```python
from build123d import *

# Parameters (mm, degrees)
SKETCH1_R          = 2.667
SKETCH1_R_2        = 3.3782
BASE_FLANGE1_DEPTH = 3.175
CHAMFER2_SIZE      = 3.175
EDGE_FLANGE1_DEPTH = 38.1
CHAMFER3_SIZE      = 3.175
SKETCH9_R          = 1.905
CUT_EXTRUDE1_DEPTH = 282.707277995
CUT_EXTRUDE2_DEPTH = 283.261385688
CUT_EXTRUDE3_DEPTH = 283.261385688


# Sheet-metal steps are written as plain solids
with BuildPart() as part:
    # Sketch1 → Base-Flange1 (new body)
    with BuildSketch(Plane(origin=(0, 0, 0), x_dir=(1, 0, 0), z_dir=(0, 1, 0))):
        Polygon((25.4, 0), (0, 0), (0, 132.588), (241.3, 132.588), (241.3, 0), (215.9, 0), (215.9, 21.463), (212.725, 24.638), (212.725, 107.188), (28.575, 107.188), (28.575, 24.638), (25.4, 21.463), align=None)
        with Locations(Location((6.35, 12.7, 0), (0, 0, 270))):
            Circle(SKETCH1_R, mode=Mode.SUBTRACT)
        with Locations(Location((19.05, 12.7, 0), (0, 0, 270))):
            Circle(SKETCH1_R, mode=Mode.SUBTRACT)
        with Locations(Location((222.25, 12.7, 0), (0, 0, 90))):
            Circle(SKETCH1_R, mode=Mode.SUBTRACT)
        with Locations(Location((234.95, 12.7, 0), (0, 0, 90))):
            Circle(SKETCH1_R, mode=Mode.SUBTRACT)
        with Locations(Location((69.85, 114.3, 0), (0, 0, 270))):
            Circle(SKETCH1_R_2, mode=Mode.SUBTRACT)
        with Locations(Location((171.45, 114.3, 0), (0, 0, 90))):
            Circle(SKETCH1_R_2, mode=Mode.SUBTRACT)
    extrude(amount=BASE_FLANGE1_DEPTH)

    # Chamfer2
    chamfer2_edges = [part.edges().sort_by_distance(p)[0] for p in [
        (0, 1.5875, -132.588),
        (241.3, 1.5875, -132.588),
        (241.3, 1.5875, 0),
        (215.9, 1.5875, 0),
        (212.725, 1.5875, -107.188),
        (28.575, 1.5875, -107.188),
        (25.4, 1.5875, 0),
        (0, 1.5875, 0),
    ]]
    chamfer(chamfer2_edges, length=CHAMFER2_SIZE)

    # Edge-Flange1 section (across the edge) → Edge-Flange1 (add)
    with BuildSketch(Plane(origin=(101.6, 0, -134.1755), x_dir=(0, 0, 1), z_dir=(1, 0, 0))):
        with BuildLine():
            Line((-3.175, 1.5875), (-3.175, 47.625))
            Line((-3.175, 47.625), (0, 47.625))
            Line((0, 47.625), (0, 1.5875))
            ThreePointArc((0, 1.5875), (0.464967985, 0.464967985), (1.5875, 0))
            Line((1.5875, 0), (1.5875, -3.175))
            ThreePointArc((1.5875, -3.175), (-1.780096045, -1.780096045), (-3.175, 1.5875))
        make_face()
    extrude(amount=EDGE_FLANGE1_DEPTH)

    # Chamfer3
    chamfer3_edges = [part.edges().sort_by_distance(p)[0] for p in [
        (101.6, -47.625, -135.763),
        (139.7, -47.625, -135.763),
    ]]
    chamfer(chamfer3_edges, length=CHAMFER3_SIZE)

    # Sketch9 → Cut-Extrude1 (cut, through all)
    with BuildSketch(Plane(origin=(0, 0, -137.3505), x_dir=(-1, 0, 0), z_dir=(0, 0, -1))):
        with Locations(Location((-120.65, -38.989, 0), (0, 0, 90))):
            Circle(SKETCH9_R)
        with Locations(Location((-120.65, -19.939, 0), (0, 0, 90))):
            Circle(SKETCH9_R)
    extrude(amount=-CUT_EXTRUDE1_DEPTH, mode=Mode.SUBTRACT)

    # Sketch10 → Cut-Extrude2 (cut, through all)
    with BuildSketch(Plane(origin=(0, 3.175, 0), x_dir=(1, 0, 0), z_dir=(0, 1, 0))):
        with BuildLine():
            Line((115.8875, 127.8255), (125.4125, 127.8255))
            ThreePointArc((125.4125, 127.8255), (127, 126.238), (125.4125, 124.6505))
            Line((125.4125, 124.6505), (115.8875, 124.6505))
            ThreePointArc((115.8875, 124.6505), (114.3, 126.238), (115.8875, 127.8255))
        make_face()
    extrude(amount=-CUT_EXTRUDE2_DEPTH, mode=Mode.SUBTRACT)

    # Sketch11 → Cut-Extrude3 (cut, through all)
    with BuildSketch(Plane(origin=(0, 3.175, 0), x_dir=(1, 0, 0), z_dir=(0, 1, 0))):
        with BuildLine():
            Line((107.95, 119.09425), (133.35, 119.09425))
            ThreePointArc((133.35, 119.09425), (135.73125, 116.713), (133.35, 114.33175))
            Line((133.35, 114.33175), (107.95, 114.33175))
            ThreePointArc((107.95, 114.33175), (105.56875, 116.713), (107.95, 119.09425))
        make_face()
    extrude(amount=-CUT_EXTRUDE3_DEPTH, mode=Mode.SUBTRACT)


solid = part.part
```
The model under review builds one solid part; all positions refer to its coordinate system, in mm. A direction names the side the tool comes from. Round coordinates to 2 decimals unless told otherwise and drop trailing zeros. Order: outer loops, then holes, each group sorted by start corner. A loop starts at its lowest first (then second) coordinate and runs counter-clockwise, first axis right, second up. Notation, with made-up numbers: (72, 44.5) -> (89, 44.5) arc R15 cw to (89, 52.5) -> close; hole circle Ø8 at (-27.75, 45). An arc over 180 degrees is marked (long way). One line per item, written item: value. Start each with the question number.
Q1. Take a section at D-D (y = -11.5). Write out the cut boundary in (x, z), and give its area (3 significant figures).
Q2. Mouldability with a two-part tool opening along X and no side actions: class faces 1 (the face through (101.6, -21, -135)), 2 (the face through (7.151, 1.565, -10.156)), 3 (the face through (120.383, 1.817, -135.918)), 4 (the face through (66.853, 1.565, -112.741)) as released by +X, released by -X, zero draft, split by the parting line, or undercut.
Q3. Take a section at B-B (z = -58). Write out the cut boundary in (x, y) (3 decimals), and give its area (3 significant figures).
Q4. Clearance check with flat-ended pins moving along their axes: pin 1 Ø1.6 at (x, y) = (121, 1.5) entering from -Z; pin 2 Ø2.5 at (x, y) = (117, 1.5) entering from -Z; pin 3 Ø3.5 at (x, y) = (83, 1) entering from +Z. State where each tip first meets the part, or that it passes through.
Q5. Wall thickness on line 1 (X direction, y = 1.3, z = -12.7); line 2 (X direction, y = 2, z = -114); line 3 (Z direction, x = 83.5, y = 0.5): over which ranges is each line inside the solid? List them lowest first.
Q6. Take a section at A-A (x = 131). Write out the cut boundary in (y, z) (1 decimal), and give its area (3 significant figures).
Q7. Machinability: for faces 5 (the face through (172.744, 1.565, -117.421)), 6 (the face through (139.7, -21, -135)), 7 (the face through (120, -25, -134.176)), which of the approach directions +Z, -Z, +X, -X, +Y, -Y give a long, thin tool a straight path to every point of the face, cutting with its end or side? Answer none if there is none.
Q8. Take a section at C-C (x = 19.05). Write out the cut boundary in (y, z) (3 decimals), and give its area (3 significant figures).
Reported:
1. outline: (101.6, -137.35) -> (139.7, -137.35) -> (139.7, -134.18) -> (101.6, -134.18) -> close
1. area: 121 mm2
2. face 1: released by -X
2. face 2: undercut
2. face 3: zero draft
2. face 4: undercut
3. outline: (0, 0) -> (28.575, 0) -> (28.575, 3.175) -> (0, 3.175) -> close; (212.725, 0) -> (241.3, 0) -> (241.3, 3.175) -> (212.725, 3.175) -> close
3. area: 181 mm2
4. pin 1: stops at z = -136.77
4. pin 2: stops at z = -136.98
4. pin 3: stops at z = -107.19
5. line 1: x = 0 to 3.68, 9.02 to 16.38, 21.72 to 25.4, 215.9 to 219.58, 224.92 to 232.28, 237.62 to 241.3
5. line 2: x = 0 to 66.49, 73.21 to 168.09, 174.81 to 241.3
5. line 3: z = -132.59 to -107.19
6. outline: (-47.6, -137.4) -> (-1.6, -137.4) arc R4.8 ccw to (3.2, -132.6) -> (3.2, -119.1) -> (0, -119.1) -> (0, -132.6) arc R1.6 cw to (-1.6, -134.2) -> (-47.6, -134.2) -> close; (0, -114.3) -> (3.2, -114.3) -> (3.2, -107.2) -> (0, -107.2) -> close
6. area: 228 mm2
7. face 5: +Y, -Y
7. face 6: -Z, +X, +Y, -Y
7. face 7: +Z, +X, -X, -Y
8. outline: (0, -132.588) -> (3.175, -132.588) -> (3.175, -15.367) -> (0, -15.367) -> close; (0, -10.033) -> (3.175, -10.033) -> (3.175, 0) -> (0, 0) -> close
8. area: 404 mm2
